Source: CAD feature listing. Evaluate the final solid. Frame: model axes, mm. A direction names the side the tool comes from. Coordinates: 2 decimals unless noted, no trailing zeros. Loops run counter-clockwise (first coordinate to the right, second up) from the corner with the lowest first, then second, coordinate; pieces in that order, holes last.
Item 1: Section query C-C, the plane x = 1. Return the cut outline in (y, z), then the cut area to 3 significant figures.
Item 2: Section query A-A, the plane y = 10. Return the cut outline in (x, z), then the cut area to 3 significant figures.
Item 3: Line query: probe 1 along Z at (x, y) = (1.45, 10); probe 2 along Y at (x, z) = (1.2, 5); probe 3 along X at (y, z) = (2, 2). Output: solid intervals per line, ascending.
Item 4: Section query D-D, the plane z = 7.5. Return the cut outline in (x, y).
Item 5: Reachability of faces 4 (the flat face through (7, 0, 2)), 5 (the flat face through (12, 3, 5)), 6 (the flat face through (-0.5, 0, 5)) from +Z, -Z, +X, -X, +Y, -Y: full face, straight path, thin tool, end or side. Return the list, or none.
Item 6: Pin query (flat end, axial travel): pin 1 Ø0.5 at (x, y) = (5, -0.5) entering from +Z; pin 2 Ø0.8 at (x, y) = (-0.5, 12) entering from -Z; pin 3 Ø5 at (y, z) = (6, 8) entering from +X. Return the tip coordinate at first contact, or that it passes through.
Item 7: Pull-direction query (Y, two-part tool) for faces 1 (the flat face through (15, 1, 5)), 2 (the cylindrical face through (0.972, 9.425, 6.386)), 3 (the flat face through (5, -1, 5)); classes: +Y half, -Y half, draft (parallel to the pull), parting line (faces both ways), or undercut.
```python
from build123d import *

# Parameters (mm, degrees)
MAIN_DEPTH                         = 10
ESQUISSE4_W                        = 2.9
ESQUISSE4_H                        = 15
MAKERBEAMFIXVERTICAL_DEPTH         = 1
ESQUISSE2_R                        = 1.5
MAKERBEAMVERTICALHOLE_DEPTH        = 2
MAKERBEAMVERTICALHOLE_DEPTH_BACK   = 16
ESQUISSE5_W                        = 15
ESQUISSE5_H                        = 2.9
MAKERBEAMFIXHORIZONTAL_DEPTH       = 1
ESQUISSE3_R                        = 1.5
MAKERBEAMHORIZONTALHOLE_DEPTH      = 2
MAKERBEAMHORIZONTALHOLE_DEPTH_BACK = 16


with BuildPart() as part:
    # Esquisse1 → Main (new body)
    with BuildSketch(Plane.XY):
        with BuildLine():
            Line((0, 0), (15, 0))
            Line((15, 0), (15, 3))
            Line((15, 3), (7, 3))
            ThreePointArc((7, 3), (4.171572875, 4.171572875), (3, 7))
            Line((3, 7), (3, 15))
            Line((3, 15), (0, 15))
            Line((0, 15), (0, 0))
        make_face()
    extrude(amount=MAIN_DEPTH)

    # Esquisse4 → MakerBeamFixVertical (add)
    with BuildSketch(Plane.ZY):
        with Locations((5, 7.5)):
            Rectangle(ESQUISSE4_W, ESQUISSE4_H)
    extrude(amount=MAKERBEAMFIXVERTICAL_DEPTH)

    # Esquisse2 → MakerBeamVerticalHole (cut, two sides)
    with BuildSketch(Plane.ZY) as makerbeamverticalhole_sk:
        with Locations((5, 10)):
            Circle(ESQUISSE2_R)
    extrude(amount=MAKERBEAMVERTICALHOLE_DEPTH, mode=Mode.SUBTRACT)
    extrude(makerbeamverticalhole_sk.sketch, amount=-MAKERBEAMVERTICALHOLE_DEPTH_BACK, mode=Mode.SUBTRACT)

    # Esquisse5 → MakerBeamFixHorizontal (add)
    with BuildSketch(Plane(origin=(0, 0, 0), x_dir=(-1, 0, 0), z_dir=(0, -1, 0))):
        with Locations((-7.5, -5)):
            Rectangle(ESQUISSE5_W, ESQUISSE5_H)
    extrude(amount=MAKERBEAMFIXHORIZONTAL_DEPTH)

    # Esquisse3 → MakerBeamHorizontalHole (cut, two sides)
    with BuildSketch(Plane.XZ) as makerbeamhorizontalhole_sk:
        with Locations((10, 5)):
            Circle(ESQUISSE3_R)
    extrude(amount=MAKERBEAMHORIZONTALHOLE_DEPTH, mode=Mode.SUBTRACT)
    extrude(makerbeamhorizontalhole_sk.sketch, amount=-MAKERBEAMHORIZONTALHOLE_DEPTH_BACK, mode=Mode.SUBTRACT)


solid = part.part
```
Verdict:
1. outline: (-1, 3.55) - (0, 3.55) - (0, 0) - (15, 0) - (15, 10) - (0, 10) - (0, 6.45) - (-1, 6.45) - close; hole circle Ø3 at (10, 5)
1. area: 146 mm2
2. outline: (0, 0) - (3, 0) - (3, 3.5) - (0, 3.5) - close; (0, 6.5) - (3, 6.5) - (3, 10) - (0, 10) - close
2. area: 21.0 mm2
3. probe 1: z = 0 to 3.5, 6.5 to 10
3. probe 2: y = -1 to 8.5, 11.5 to 15
3. probe 3: x = 0 to 15
4. outline: (0, 0) - (15, 0) - (15, 3) - (7, 3) arc R4 cw to (3, 7) - (3, 15) - (0, 15) - close
5. face 4: -Z, +X, -X, -Y
5. face 5: +Z, -Z, +X, +Y
5. face 6: +Z, -Z, -X, -Y
6. pin 1: stops at z = 6.45
6. pin 2: stops at z = 3.55
6. pin 3: stops at x = 5.06
7. face 1: draft
7. face 2: undercut
7. face 3: -Y half
